Study the drawing (mm; zero at the part's minimum x, y, z) and answer. Give positions to 0.01 mm unless a question says otherwise; leave off trailing zeros. Order: outer loops, then holes, each group sorted by start corner. A loop starts at its lowest first (then second) coordinate and runs counter-clockwise, first axis right, second up. Notation, with made-up numbers: (-34, 47) - (-17, 47) arc R17 cw to (-17, 59) - close; hole circle Ø8 at (17, 45.25). An arc over 180 degrees is marked (long way). Write each question's results on one line, items separated by ' | '. Start each with the question number.
Q1. Find section D-D on x = 1.25. Give the vertices of the cut face in (y, z) (1 decimal), and give its area (3 significant figures).
Q2. Find the intervals of material crossed by line 1 along X through (y, z) = (5.75, 0.5); line 2 along Y through (x, z) = (3.25, 2.25) (1 decimal); line 3 along Y through (x, z) = (4.75, 2.25) (1 decimal), in increasing order. Write a range as from..to.
Q3. Find section B-B on x = 5.5. Give the vertices of the cut face in (y, z).
Q4. Find section A-A on z = 4. Give the vertices of the cut face in (x, y) (1 decimal).
Q5. For a pull along Y with two mould halves and no side action, classify the marked faces 1, 2 and 3 as +Y half, -Y half, draft (parallel to the pull), parting line (faces both ways), or undercut.
Q6. Find section C-C on y = 5.75. Give the vertices of the cut face in (x, z).
Q7. Flat-ended cylindrical pins translate along their axes: P1, Ø3.5, axis at x = 5, y = 5.77, coming from the +Z side; P2, Ø2, axis at x = 8.5, z = 3, coming from the +Y side (1 decimal). Find the tip coordinate at first contact, or state that the pin passes through.
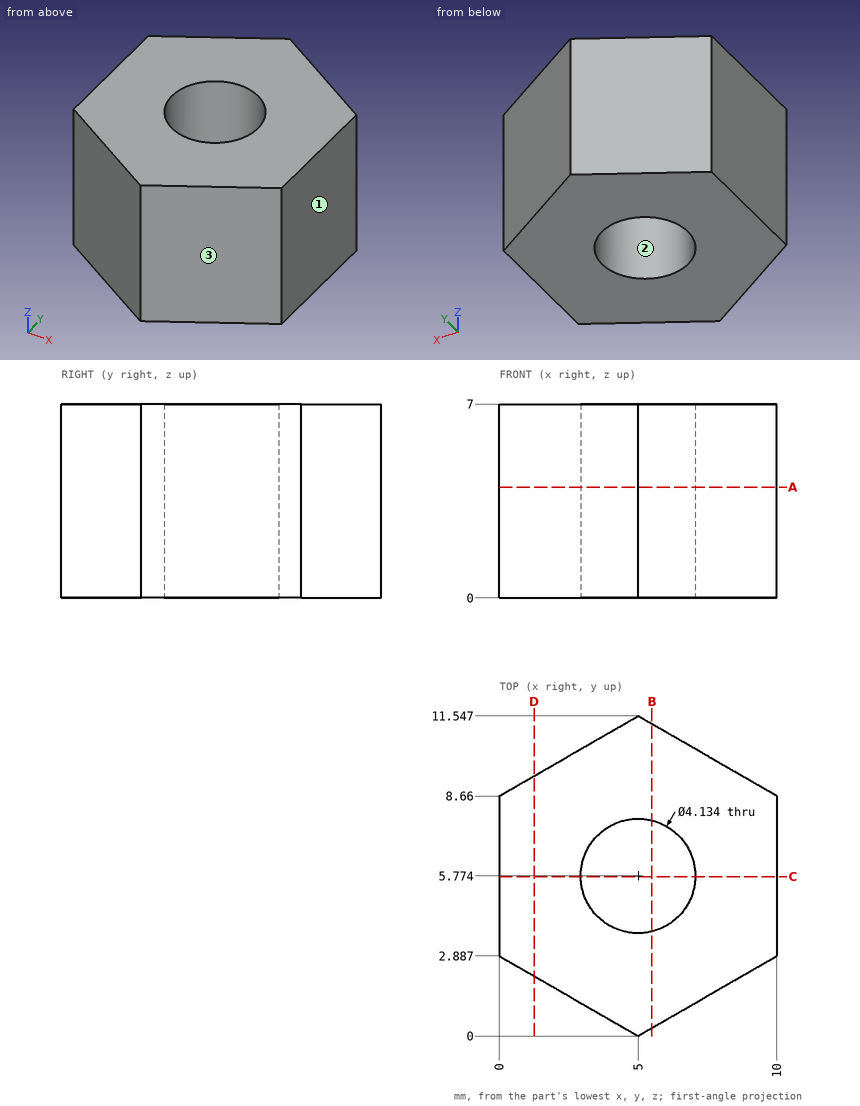
Working result:
1) outline: (2.2, 0) - (9.4, 0) - (9.4, 7) - (2.2, 7) - close | area: 50.5 mm²
2) line 1: 0..2.93, 7.07..10 | line 2: 1..4.7, 6.9..10.5 | line 3: 0.1..3.7, 7.8..11.4
3) outline: (0.29, 0) - (3.77, 0) - (3.77, 7) - (0.29, 7) - close; (7.78, 0) - (11.26, 0) - (11.26, 7) - (7.78, 7) - close
4) outline: (0, 2.9) - (5, 0) - (10, 2.9) - (10, 8.7) - (5, 11.5) - (0, 8.7) - close; hole circle Ø4.1 at (5, 5.8)
5) face 1: draft | face 2: undercut | face 3: -Y half
6) outline: (0, 0) - (2.93, 0) - (2.93, 7) - (0, 7) - close; (7.07, 0) - (10, 0) - (10, 7) - (7.07, 7) - close
7) P1: through | P2: y = 10.1
